```python
from build123d import *

# Parameters (mm, degrees)
EXTRUDE_1_DEPTH     = 15
SKETCH_2_R          = 1
CUT_EXTRUDE_1_DEPTH = 2
SKETCH_3_R          = 1
CUT_EXTRUDE_2_DEPTH = 2


with BuildPart() as part:
    # 草图1 → 凸台-拉伸1 (new body)
    with BuildSketch(Plane.XY):
        Polygon((0, 0), (-15, 0), (-15, 1), (-1, 1), (-1, 15), (0, 15), align=None)
    extrude(amount=EXTRUDE_1_DEPTH)

    # 草图2 → 切除-拉伸1 (cut, through all)
    with BuildSketch(Plane.ZY.offset(1)):
        with Locations((7.5, 8.288332676)):
            Circle(SKETCH_2_R)
    extrude(amount=-CUT_EXTRUDE_1_DEPTH, mode=Mode.SUBTRACT)

    # 草图3 → 切除-拉伸2 (cut, through all)
    with BuildSketch(Plane(origin=(0, 1, 0), x_dir=(1, 0, 0), z_dir=(0, 1, 0))):
        with Locations((-8, -7.011984534)):
            Circle(SKETCH_3_R)
    extrude(amount=-CUT_EXTRUDE_2_DEPTH, mode=Mode.SUBTRACT)


solid = part.part
```
The listing builds one solid part. Answer for the finished solid, in the listing's coordinates (mm). A direction names the side the tool comes from. Give positions to 0.01 mm unless a question says otherwise; leave off trailing zeros. Order: outer loops, then holes, each group sorted by start corner. A loop starts at its lowest first (then second) coordinate and runs counter-clockwise, first axis right, second up. Notation, with made-up numbers: M 24,-29.75 L 77,-29.75 A20 cw 77,0.25 Z; hole C 32.25,8 d8. An arc over 180 degrees is marked long. Put each result on its own line as item: value. Start each with the question number.
Item 1: Which of the six approach directions +Z, -Z, +X, -X, +Y, -Y give full straight-line access (tool end or side, diameter ignored) to faces 1 (the face through (-15, 0.5, 7.4)), 2 (the face through (-1, 9.5, 7.4))?
Item 2: For a pull along X with two mould halves and no side action, classify faces 3 (the face through (-6.5, 1, 7.4)), 4 (the face through (0, 6, 7)), 5 (the face through (-8.217, 0.507, 7.988)) as +X half, -X half, draft (parallel to the pull), parting line (faces both ways), or undercut.
Item 3: Find the intervals of material crossed by line 1 along Z through (x, y) = (-8, 0.6); line 2 along X through (y, z) = (8.5, 13); line 3 along Y through (x, z) = (-11.5, 12.75), in increasing order.
Item 4: The part is cut by section B-B, the plane z = 7.5. Determine the outline of the cut face in (x, y), and give its area (3 significant figures).
Item 5: The part is cut by section A-A, the plane x = -8. Determine the outline of the cut face in (y, z).
Item 6: Flat-ended cylindrical pins translate along their axes: P1, Ø1.5, axis at x = -12, z = 13.5, coming from the +Y side; P2, Ø5, axis at x = -5.5, z = 10.5, coming from the -Y side; P3, Ø4, axis at y = 6, z = 1.5, coming from the -X side. Find the tip coordinate at first contact, or state that the pin passes through.
Item 7: The part is cut by section C-C, the plane y = 10.5. Determine the outline of the cut face in (x, z), and give its area (3 significant figures).
Item 8: The part is cut by section D-D, the plane x = -10.5. Determine the outline of the cut face in (y, z), and give its area (3 significant figures).
Answer key:
1. face 1: +Z, -Z, -X, +Y, -Y
1. face 2: +Z, -Z, -X, +Y
2. face 3: draft
2. face 4: +X half
2. face 5: undercut
3. line 1: z = 0 to 6.01, 8.01 to 15
3. line 2: x = -1 to 0
3. line 3: y = 0 to 1
4. outline: M -15,0 L -8.87,0 L -8.87,1 L -15,1 Z; M -7.13,0 L 0,0 L 0,7.29 L -1,7.29 L -1,1 L -7.13,1 Z; M -1,9.29 L 0,9.29 L 0,15 L -1,15 Z
4. area: 25.3 mm²
5. outline: M 0,0 L 1,0 L 1,6.01 L 0,6.01 Z; M 0,8.01 L 1,8.01 L 1,15 L 0,15 Z
6. P1: stops at y = 1
6. P2: stops at y = 0
6. P3: stops at x = -1
7. outline: M -1,0 L 0,0 L 0,15 L -1,15 Z
7. area: 15.0 mm²
8. outline: M 0,0 L 1,0 L 1,15 L 0,15 Z
8. area: 15.0 mm²
